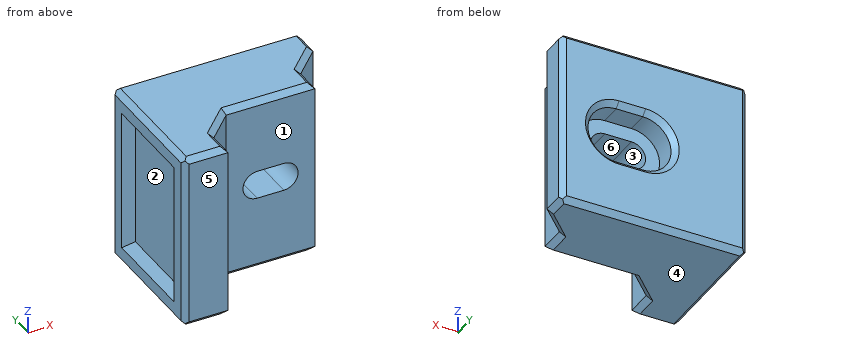
Autodesk Inventor part; units mm, degrees
ref_plane "YZ Plane" through (0, 0, 0) normal (1, 0, 0) x (0, 1, 0)
ref_plane "XZ Plane" through (0, 0, 0) normal (0, 1, 0) x (-1, 0, 0)
ref_plane "XY Plane" through (0, 0, 0) normal (0, 0, 1) x (1, 0, 0)
sketch "Sketch1" plane through (0, 0, 0) normal (0, 0, 1) x (1, 0, 0)
  line L0 (0, 0) -> (5, 0)
  line L1 (5, 0) -> (5, 3)
  line L2 (5, 3) -> (8, 6)
  line L3 (8, 6) -> (18, 6)
  line L4 (21, 15) -> (0, 15)
  line L5 (0, 15) -> (0, 0)
  line L6 (18, 6) -> (18, 9)
  line L7 (18, 9) -> (21, 12)
  line L8 (21, 12) -> (21, 15)
  dimension "d0" = 45
  dimension "d2" = 5
  dimension "d4" = 10
  dimension "d6" = 3
  dimension "d7" = 3
  dimension "d8" = 3
  dimension "d25" = 3
extrude "Extrusion1" add sketch "Sketch1" along normal blind 20
sketch "Sketch2" plane through (0, 15, 0) normal (0, 1, 0) x (1, 0, 0)
  line L0 (9.9, -10) -> (16.1, -10) construction
  line L1 (11.5, -11.6) -> (14.5, -11.6)
  line L2 (14.5, -8.4) -> (11.5, -8.4)
  arc A0 (11.5, -8.4) -> (11.5, -11.6) centre (11.5, -10) ccw
  arc A1 (14.5, -11.6) -> (14.5, -8.4) centre (14.5, -10) ccw
  line L3 (11.5, -10) -> (14.5, -10) construction
  line L4 (11.5, -13.175) -> (14.5, -13.175)
  line L5 (14.5, -6.825) -> (11.5, -6.825)
  arc A2 (11.5, -6.825) -> (11.5, -13.175) centre (11.5, -10) ccw
  arc A3 (14.5, -13.175) -> (14.5, -6.825) centre (14.5, -10) ccw
  line L6 (8, 0) -> (18, 0) construction
  line L7 (18, 0) -> (18, -20) construction
  line L8 (8, -20) -> (18, -20) construction
  line L9 (8, 0) -> (8, -20) construction
  point P0 (13, -10)
  point P1 (8.325, -10)
  point P2 (13, -20)
  point P3 (8, -10)
  dimension "d11" = 3.2
  dimension "d16" = 6.35
  dimension "d24" = 3
extrude "Extrusion2" cut sketch "Sketch2" against normal through all contours A0 L2 A1 L1
extrude "Extrusion3" cut sketch "Sketch2" against normal blind 3 contours A0 L2 A1 L1 | A2 L5 A3 L4
sketch "Sketch3" plane through (0, 0, 0) normal (-1, 0, 0) x (0, 0, 1)
  line L0 (0, 15) -> (0, 0) construction
  line L1 (0, 0) -> (20, 0) construction
  line L2 (20, 15) -> (20, 0) construction
  line L3 (0, 15) -> (20, 15) construction
  line L4 (17, 12) -> (17, 3)
  line L5 (17, 3) -> (3, 3)
  line L6 (3, 3) -> (3, 12)
  line L7 (3, 12) -> (17, 12)
  dimension "d26" = 3
extrude "Extrusion4" cut sketch "Sketch3" against normal blind 1
chamfer "Chamfer1" distance 0.6 angle 45 25 edges at (10.5, 15, 20) (10.5, 15, 0) (0, 15, 10) (0, 7.5, 20) (0, 7.5, 0) (0, 0, 10) (2.5, 0, 20) (2.5, 0, 0) (19.5, 10.5, 20) (18, 7.5, 20) (13, 6, 20) (6.5, 4.5, 20) (5, 1.5, 20) (5, 1.5, 0) (6.5, 4.5, 0) (13, 6, 0) (18, 7.5, 0) (19.5, 10.5, 0) (17.675, 15, 10) (13, 15, 13.175) (8.325, 15, 10) (13, 15, 6.825) (21, 13.5, 20) (21, 13.5, 0) (21, 15, 10)
chamfer "Chamfer2" distance 1 angle 45 4 edges at (0, 7.5, 3) (0, 12, 10) (0, 7.5, 17) (0, 3, 10)
equation "\"d7\" = d6"
equation "\"d8\" = d7"
equation "\"d25\" = d7"
Source: CAD feature listing. Evaluate the final solid. Frame: model axes, mm. Face numbers are marked on the shaded views. A direction names the side the tool comes from. Give positions to 0.01 mm unless a question says otherwise; leave off trailing zeros. Loops run counter-clockwise (first coordinate to the right, second up) from the corner with the lowest first, then second, coordinate; pieces in that order, holes last. Notation, with made-up numbers: M 25.25,52.25 L 48.25,52.25 A36 ccw 48.25,90.25 Z; hole C 26.25,-38 d4. An arc over 180 degrees is marked long. Put each result on its own line as item: value.
Q1. Mould query, pull axis Z, two halves, no side actions, for the marked faces 4, 5 and 6. Classes: released by +Z, released by -Z, zero draft, split by the parting line, or undercut.
Response values:
face 4: released by -Z
face 5: zero draft
face 6: undercut
Q2. Section D-D (x = 6.25). Return the cut outline in (y, z), and give its area (3 significant figures).
Response values:
outline: M 4.25,0.6 L 5.1,0 L 14.4,0 L 15,0.6 L 15,19.4 L 14.4,20 L 5.1,20 L 4.25,19.4 Z
area: 214 mm²
Q3. Section C-C (y = 1). Return the cut outline in (x, z), and give its area (3 significant figures).
Response values:
outline: M 0,0.6 L 0.6,0 L 4.4,0 L 5,0.6 L 5,19.4 L 4.4,20 L 0.6,20 L 0,19.4 Z
area: 99.3 mm²
Q4. Reachability of the marked faces 1, 2 and 3 from +Z, -Z, +X, -X, +Y, -Y: full face, straight path, thin tool, end or side. Return the list, or none.
Response values:
face 1: +Z, -Z, +X, -Y
face 2: -X
face 3: +Y, -Y
Q5. Pin query (flat end, axial travel): P1, Ø3.5, axis at y = 1.5, z = 12.5, coming from the +X side; P2, Ø1.5, axis at y = 7.5, z = 11.5, coming from the +X side; P3, Ø11, axis at x = 14, z = 10, coming from the -Y side. Return the tip coordinate at first contact, or that it passes through.
Response values:
P1: stops at x = 5.25
P2: stops at x = 18
P3: stops at y = 6
Q6. Line query: probe 1 along Z at (x, y) = (13, 14) (3 decimals); probe 2 along Y at (x, z) = (12.75, 13); probe 3 along Z at (x, y) = (13.5, 9). Output: solid intervals per line, ascending. Write a range as [from, to].
Response values:
probe 1: z = [0, 6.825], [13.175, 20]
probe 2: y = [6, 12]
probe 3: z = [0, 8.4], [11.6, 20]
